from build123d import *

# Parameters (mm, degrees)
SKETCH_R           = 2.6
PAD_DEPTH          = 9.5
SKETCH001_R        = 1.6
POCKET_DEPTH       = 10.001
POCKET_FACE8_W     = 45
POCKET_FACE8_H     = 9.5
POCKET_FACE8_R     = 1.6
POCKET001_DEPTH    = 1.5
PAD001_DEPTH       = 45
PAD001_FACE15_R    = 1.6
POCKET002_DEPTH    = 1.501
POCKET003_DEPTH    = 9.501
FILLET_R           = 1.5
POCKET004_DEPTH    = 45.001
POCKET004_FACE12_W = 45
POCKET004_FACE12_H = 9.5
POCKET004_FACE12_R = 1.6
PAD002_DEPTH       = 1.5
FILLET001_R        = 3
FILLET002_R        = 1


with BuildPart() as part:
    # Sketch → Pad (new body)
    with BuildSketch(Plane.XY):
        with BuildLine():
            Line((22.5, -24.6), (-22.5, -24.6))
            Line((-22.5, -24.6), (-22.5, -14.6))
            Line((-22.5, -14.6), (-15.5, -14.6))
            Line((-15.5, -14.6), (-4.77656, 2.923094))
            ThreePointArc((4.77656, 2.923094), (0, 5.6), (-4.77656, 2.923094))
            Line((15.5, -14.6), (4.77656, 2.923094))
            Line((15.5, -14.6), (22.5, -14.6))
            Line((22.5, -14.6), (22.5, -24.6))
        make_face()
        Circle(SKETCH_R, mode=Mode.SUBTRACT)
    extrude(amount=PAD_DEPTH)

    # Sketch001 (on Face1 of Pad) → Pocket (cut, through all)
    with BuildSketch(Plane(origin=(0, -14.6, 0), x_dir=(-1, 0, 0), z_dir=(0, 1, 0))):
        with Locations((-18.865231, 4.75)):
            Circle(SKETCH001_R)
        with Locations((18.865231, 4.75)):
            Circle(SKETCH001_R)
    extrude(amount=-POCKET_DEPTH, mode=Mode.SUBTRACT)

    # Pocket Face8 → Pocket001 (cut)
    with BuildSketch(Plane(origin=(0, -24.6, 4.75), x_dir=(-1, 0, 0), z_dir=(0, -1, 0))):
        Rectangle(POCKET_FACE8_W, POCKET_FACE8_H)
        with Locations((-18.865231, 0)):
            Circle(POCKET_FACE8_R, mode=Mode.SUBTRACT)
        with Locations((18.865231, 0)):
            Circle(POCKET_FACE8_R, mode=Mode.SUBTRACT)
    extrude(amount=-POCKET001_DEPTH, mode=Mode.SUBTRACT)

    # Sketch002 (on Face9 of Pocket001) → Pad001 (join)
    with BuildSketch(Plane(origin=(-22.5, 0, 0), x_dir=(0, -1, 0), z_dir=(-1, 0, 0))):
        Polygon((23.1, 9.5), (23.1, 0), (24.6, 2.25), (24.6, 7.25), align=None)
    extrude(amount=-PAD001_DEPTH)

    # Pad001 Face15 → Pocket002 (cut, through all)
    with BuildSketch(Plane(origin=(18.865231, -23.1, 4.75), x_dir=(1, 0, 0), z_dir=(0, 1, 0))):
        Circle(PAD001_FACE15_R)
    extrude(amount=-POCKET002_DEPTH, mode=Mode.SUBTRACT)

    # Sketch003 (on Face3 of Pocket002) → Pocket003 (cut, through all)
    with BuildSketch(Plane(origin=(0, 0, 0), x_dir=(1, 0, 0), z_dir=(0, 0, -1))):
        Polygon((0, 5.6), (-9.791367, 21.6), (9.791367, 21.6), align=None)
    extrude(amount=-POCKET003_DEPTH, mode=Mode.SUBTRACT)

    # Fillet
    fillet_edges = [part.edges().sort_by_distance(p)[0] for p in [
        (9.791367, -21.6, 4.75),
        (-9.791367, -21.6, 4.75),
        (0, -5.6, 4.75),
    ]]
    fillet(fillet_edges, radius=FILLET_R)

    # Fillet Face19 → Pocket004 (cut, through all)
    with BuildSketch(Plane(origin=(22.5, -23.772414, 4.75), x_dir=(0, -1, 0), z_dir=(1, 0, 0))):
        Polygon((-0.672414, 4.75), (-0.672414, -4.75), (0.827586, -2.5), (0.827586, 2.5), align=None)
    extrude(amount=-POCKET004_DEPTH, mode=Mode.SUBTRACT)

    # Pocket004 Face12 → Pad002 (add)
    with BuildSketch(Plane(origin=(0, -23.1, 4.75), x_dir=(-1, 0, 0), z_dir=(0, -1, 0))):
        Rectangle(POCKET004_FACE12_W, POCKET004_FACE12_H)
        with Locations((18.865231, 0)):
            Circle(POCKET004_FACE12_R, mode=Mode.SUBTRACT)
        with Locations((-18.865231, 0)):
            Circle(POCKET004_FACE12_R, mode=Mode.SUBTRACT)
    extrude(amount=PAD002_DEPTH)

    # Fillet001
    fillet001_edges = [part.edges().sort_by_distance(p)[0] for p in [
        (22.5, -18.85, 9.5),
        (22.5, -18.85, 0),
        (-22.5, -18.85, 9.5),
        (-22.5, -18.85, 0),
    ]]
    fillet(fillet001_edges, radius=FILLET001_R)

    # Fillet002
    fillet002_edges = [part.edges().sort_by_distance(p)[0] for p in [
        (15.5, -14.6, 4.75),
        (-15.5, -14.6, 4.75),
    ]]
    fillet(fillet002_edges, radius=FILLET002_R)


solid = part.part
The model under review builds one solid part; all positions refer to its coordinate system, in mm. A direction names the side the tool comes from. Round coordinates to 2 decimals unless told otherwise and drop trailing zeros. Loops run counter-clockwise (first coordinate to the right, second up) from the corner with the lowest first, then second, coordinate; pieces in that order, holes last. Notation, with made-up numbers: (-8.75, 87.5) -> (26.25, 87.5) arc R23 ccw to (26.25, 116.5) -> close; hole circle Ø5 at (27, -31.5). An arc over 180 degrees is marked (long way). One line per question, with ' | ' between items. Start each with the question number.
Item 1: Draft analysis for pull direction X (two halves, no side actions). For faces 6 (the face through (4.89, -13.59, 4.68)), 7 (the face through (-10.065, -5.719, 4.684)), 8 (the face through (0.021, -6.974, 4.816)), 9 (the face through (0, -24.6, 5)), state which applies: +X half, -X half, draft (parallel to the pull), parting line (faces both ways), or undercut.
Item 2: Add section C-C, the plane y = -16. Write out the cut boundary in (x, z), then the cut area to 3 significant figures.
Item 3: Add section B-B, the plane x = 0. Write out the cut boundary in (y, z).
Item 4: For pin 1 (2 mm diameter, centred on y = -1.5, z = 2, fed in from +X); pin 2 (5 mm diameter, centred on x = -18.87, z = 4.75, fed in from +Y); pin 3 (8 mm diameter, centred on x = -11.5, y = -2, fed in from +Z); pin 4 (2 mm diameter, centred on y = 2.5, z = 4.5, fed in from -X), all flat-tipped, find the tip position at first contact; note any pin that passes through.
Item 5: Add section A-A, the plane z = 4.75. Write out the cut boundary in (x, y).
Item 6: Wall thickness on line 1 along X through (y, z) = (-22.5, 4.75); line 2 along Y through (x, z) = (0, 4); line 3 along X through (y, z) = (-23, 4.25): over which ranges is each line inside the solid? List them lowest first. Write a range as [from, to].
Item 7: Add section D-D, the plane z = 1.25. Write out the cut boundary in (x, y), then the cut area to 3 significant figures.
Item 8: Machinability: for faces 1 (the face through (-21.64, -19.53, 0.9)), 2 (the face through (-4.787, -13.422, 4.684)), 3 (the face through (21, -14.6, 5)), 4 (the face through (-21, -14.6, 5)), 5 (the face through (22.5, -20, 5)), which of the approach directions +Z, -Z, +X, -X, +Y, -Y give a long, thin tool a straight path to every point of the face, cutting with its end or side? Answer none if there is none.
Return value:
1) face 6: undercut | face 7: -X half | face 8: undercut | face 9: draft
2) outline: (-22.5, 3) arc R3 ccw to (-19.5, 0) -> (-6.36, 0) -> (-6.36, 9.5) -> (-19.5, 9.5) arc R3 ccw to (-22.5, 6.5) -> close; (6.36, 0) -> (19.5, 0) arc R3 ccw to (22.5, 3) -> (22.5, 6.5) arc R3 ccw to (19.5, 9.5) -> (6.36, 9.5) -> close; hole circle Ø3.2 at (-18.87, 4.75); hole circle Ø3.2 at (18.87, 4.75) | area: 283 mm2
3) outline: (-24.6, 0) -> (-21.6, 0) -> (-21.6, 9.5) -> (-24.6, 9.5) -> close; (-6.97, 0) -> (-2.6, 0) -> (-2.6, 9.5) -> (-6.97, 9.5) -> close; (2.6, 0) -> (5.6, 0) -> (5.6, 9.5) -> (2.6, 9.5) -> close
4) pin 1: stops at x = 8.1 | pin 2: stops at y = -14.6 | pin 3: stops at z = 9.5 | pin 4: stops at x = -5.65
5) outline: (-22.5, -24.6) -> (-20.47, -24.6) -> (-20.47, -14.6) -> (-22.5, -14.6) -> close; (-17.27, -24.6) -> (17.27, -24.6) -> (17.27, -14.6) -> (16.06, -14.6) arc R1 cw to (15.21, -14.12) -> (4.78, 2.92) arc R5.6 ccw to (-4.78, 2.92) -> (-15.21, -14.12) arc R1 cw to (-16.06, -14.6) -> (-17.27, -14.6) -> close; (20.47, -24.6) -> (22.5, -24.6) -> (22.5, -14.6) -> (20.47, -14.6) -> close; hole (-8.39, -19.32) arc R1.5 ccw to (-7.11, -21.6) -> (7.11, -21.6) arc R1.5 ccw to (8.39, -19.32) -> (1.28, -7.69) arc R1.5 ccw to (-1.28, -7.69) -> close; hole circle Ø5.2 at (0, 0)
6) line 1: x = [-22.5, -20.47], [-17.27, 17.27], [20.47, 22.5] | line 2: y = [-24.6, -21.6], [-6.97, -2.6], [2.6, 5.6] | line 3: x = [-22.5, -20.39], [-17.35, 17.35], [20.39, 22.5]
7) outline: (-21.94, -24.6) -> (21.94, -24.6) -> (21.94, -14.6) -> (16.06, -14.6) arc R1 cw to (15.21, -14.12) -> (4.78, 2.92) arc R5.6 ccw to (-4.78, 2.92) -> (-15.21, -14.12) arc R1 cw to (-16.06, -14.6) -> (-21.94, -14.6) -> close; hole (-8.39, -19.32) arc R1.5 ccw to (-7.11, -21.6) -> (7.11, -21.6) arc R1.5 ccw to (8.39, -19.32) -> (1.28, -7.69) arc R1.5 ccw to (-1.28, -7.69) -> close; hole circle Ø5.2 at (0, 0) | area: 639 mm2
8) face 1: -Z, -X, +Y, -Y | face 2: +Z, -Z | face 3: +Z, -Z, +X, +Y | face 4: +Z, -Z, -X, +Y | face 5: +Z, -Z, +X, +Y, -Y
